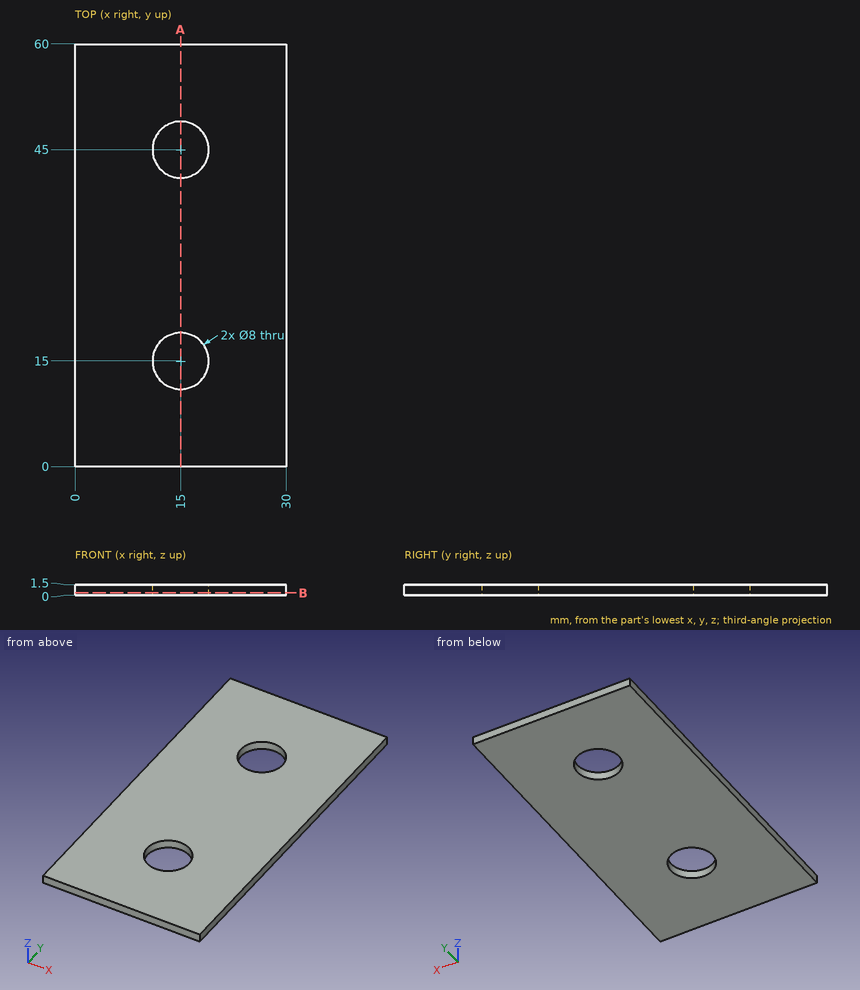
Drawing for the job (mm, zero at the part's lowest x, y, z). Give positions to 0.01 mm unless a question says otherwise; leave off trailing zeros. Order: outer loops, then holes, each group sorted by start corner. A loop starts at its lowest first (then second) coordinate and runs counter-clockwise, first axis right, second up. Notation, with made-up numbers: M 60,38.5 L 73,38.5 A33 ccw 73,74.5 Z; hole C -20.5,38.25 d7. An arc over 180 degrees is marked long. Write item = value, one per line. Start each with the question number.
(1) Slice it at A-A on x = 15. Write the cut outline in (y, z), plus the area to 3 significant figures.
(2) Probe L1, parallel to Y at x = 15, z = 0.75; L2, parallel to Y at x = 18.25, z = 1.2; L3, parallel to X at y = 42, z = 0.55 (1 decimal). List the from-to ranges inside material, lowest first. Write a range as [from, to].
(3) Pin check, flat tip, straight feed: pin 1 Ø5 at (x, y) = (15, 15) entering from -Z. Stop position of the tip, or through.
(4) Slice it at B-B on z = 0.35. Write the cut outline in (x, y), plus the area to 3 significant figures.
Responses:
q1.outline = M 0,0 L 11,0 L 11,1.5 L 0,1.5 Z; M 19,0 L 41,0 L 41,1.5 L 19,1.5 Z; M 49,0 L 60,0 L 60,1.5 L 49,1.5 Z
q1.area = 66.0 mm2
q2.L1 = [0, 11], [19, 41], [49, 60]
q2.L2 = [0, 12.67], [17.33, 42.67], [47.33, 60]
q2.L3 = [0, 12.4], [17.6, 30]
q3.pin_1 = through
q4.outline = M 0,0 L 30,0 L 30,60 L 0,60 Z; hole C 15,15 d8; hole C 15,45 d8
q4.area = 1,700 mm2
